from build123d import *

# Parameters (mm, degrees)
F0_R     = 50.8
F0_R_2   = 9.525
F1_DEPTH = 25.4
F2_R     = 44.45
F2_R_2   = 9.525
F3_DEPTH = 12.7
F4_R     = 4.7625
F5_DEPTH = 12.701
F6_SIZE  = 0.508


with BuildPart() as f1:
    # F0 (on Front) → F1 (new body)
    with BuildSketch(Plane.XZ):
        Circle(F0_R)
        Circle(F0_R_2, mode=Mode.SUBTRACT)
    extrude(amount=F1_DEPTH)

    # F2 (on face) → F3 (cut)
    with BuildSketch(Plane.XZ.offset(25.4)):
        Circle(F2_R)
        Circle(F2_R_2, mode=Mode.SUBTRACT)
    extrude(amount=-F3_DEPTH, mode=Mode.SUBTRACT)

    # F4 (on face) → F5 (cut, through all)
    with BuildSketch(Plane.XZ.offset(12.7)):
        with Locations((-26.851716639, 9.7732255955)):
            Circle(F4_R)
        with Locations((0, 28.575)):
            Circle(F4_R)
        with Locations((27.2524618676, 8.5926682208)):
            Circle(F4_R)
        with Locations((16.3899466687, -23.4072696656)):
            Circle(F4_R)
        with Locations((-17.3953578339, -22.6700716988)):
            Circle(F4_R)
    extrude(amount=-F5_DEPTH, mode=Mode.SUBTRACT)

    # F6
    f6_edges = [f1.edges().sort_by_distance(p)[0] for p in [
        (-44.45, -25.4, 0),
        (-4.7625, -12.7, 28.575),
        (-31.614217, -12.7, 9.773226),
        (-9.525, -12.7, 0),
        (-22.157858, -12.7, -22.670072),
        (-50.8, 0, 0),
        (11.627447, -12.7, -23.40727),
        (22.489962, -12.7, 8.592668),
        (-50.8, -25.4, 0),
        (-4.7625, 0, 28.575),
        (-31.614217, 0, 9.773226),
        (-22.157858, 0, -22.670072),
        (11.627447, 0, -23.40727),
        (22.489962, 0, 8.592668),
        (-9.525, 0, 0),
    ]]
    chamfer(f6_edges, length=F6_SIZE)


solid = f1.part
The model under review builds one solid part; all positions refer to its coordinate system, in mm. Round coordinates to 2 decimals unless told otherwise and drop trailing zeros. Order: outer loops, then holes, each group sorted by start corner. A loop starts at its lowest first (then second) coordinate and runs counter-clockwise, first axis right, second up. Notation, with made-up numbers: (47, 14) -> (70, 14) arc R24 ccw to (70, 28) -> close; hole circle Ø9 at (-4.5, 54). An arc over 180 degrees is marked (long way). Use CSV: the item, a comma, the result in double quotes. Start each with the question number.
(1) Mouldability with a two-part tool opening along Z and no side actions: class faces 1 (the face through (23.473, -6.432, 5.695)), 2 (the face through (10.5, 0, 0.7)), 3 (the face through (-7.559, -6.268, -5.796)), 4 (the face through (-11.012, -12.529, -49.592)) as pulls with the +Z half, pulls with the -Z half, needs draft (parallel to the pull), parting line crosses it, or undercut.
(2) Insertion check: pin 1 (8.5 mm diameter, centred on x = -17.4, z = -22.67, fed in from -Y); pin 2 (12 mm diameter, centred on y = -16.5, z = -38.5, fed in from +X); pin 3 (12 mm diameter, centred on y = -10, z = 32.5, fed in from -X); pin 4 (5 mm diameter, centred on y = -9, z = -7, fed in from +X). Each pin has a flat end and moves straight along its axis. Give the tip position at first contact, or say it passes through.
(3) Wall thickness on probe 1 along Z at (x, y) = (0, -7.5) (1 decimal); probe 2 along Z at (x, y) = (0, -18.75); probe 3 along X at (y, z) = (-11.25, 12): over which ranges is each line inside the solid? List them lowest first. Write a range as from..to.
(4) Consider section D-D on y = -15.75. Write out the cut boundary in (x, z), and give its area (3 significant figures).
(5) Consider section A-A on z = 0. Write out the cut boundary in (x, y) (3 decimals), and give its area (3 significant figures).
(6) Consider section B-B on x = 0. State how many separate pieces and enclosed holes the cut face has, and give its area (3 significant figures).
Responses:
1,face 1,"undercut"
1,face 2,"needs draft"
1,face 3,"undercut"
1,face 4,"parting line crosses it"
2,pin 1,"through"
2,pin 2,"x = 39.04"
2,pin 3,"x = -43.34"
2,pin 4,"x = 50.6"
3,probe 1,"-50.8..-9.5, 9.5..23.8, 33.3..50.8"
3,probe 2,"-50.8..-44.45, 44.45..50.8"
3,probe 3,"-49.36..-31.06, -22.64..23.93, 30.58..49.36"
4,outline,"circle Ø101.6 at (0, 0); hole circle Ø88.9 at (0, 0)"
4,area,"1,900 mm²"
5,outline,"(-50.8, -24.892) -> (-50.292, -25.4) -> (-44.958, -25.4) -> (-44.45, -24.892) -> (-44.45, -12.7) -> (-10.033, -12.7) -> (-9.525, -12.192) -> (-9.525, -0.508) -> (-10.033, 0) -> (-50.292, 0) -> (-50.8, -0.508) -> close; (9.525, -12.192) -> (10.033, -12.7) -> (44.45, -12.7) -> (44.45, -24.892) -> (44.958, -25.4) -> (50.292, -25.4) -> (50.8, -24.892) -> (50.8, -0.508) -> (50.292, 0) -> (10.033, 0) -> (9.525, -0.508) -> close"
5,area,"1,210 mm²"
6,separate pieces,"3"
6,enclosed holes,"0"
6,area,"1,090 mm²"
